```python
from build123d import *

# Parameters (mm, degrees)
SKETCH_R     = 14.5
PAD_DEPTH    = 35
SKETCH001_R  = 13.25
POCKET_DEPTH = 30
FILLET_R     = 1
FILLET001_R  = 1.2


with BuildPart() as part:
    # Sketch → Pad (new body)
    with BuildSketch(Plane.XY):
        Circle(SKETCH_R)
    extrude(amount=PAD_DEPTH)

    # Sketch001 (on Face3 of Pad) → Pocket (cut)
    with BuildSketch(Plane.XY.offset(35)):
        Circle(SKETCH001_R)
    extrude(amount=-POCKET_DEPTH, mode=Mode.SUBTRACT)

    # Fillet
    fillet_edges = [part.edges().sort_by_distance(p)[0] for p in [
        (-14.5, 0, 0),
    ]]
    fillet(fillet_edges, radius=FILLET_R)

    # Fillet001
    fillet001_edges = [part.edges().sort_by_distance(p)[0] for p in [
        (-14.5, 0, 35),
    ]]
    fillet(fillet001_edges, radius=FILLET001_R)


solid = part.part
```
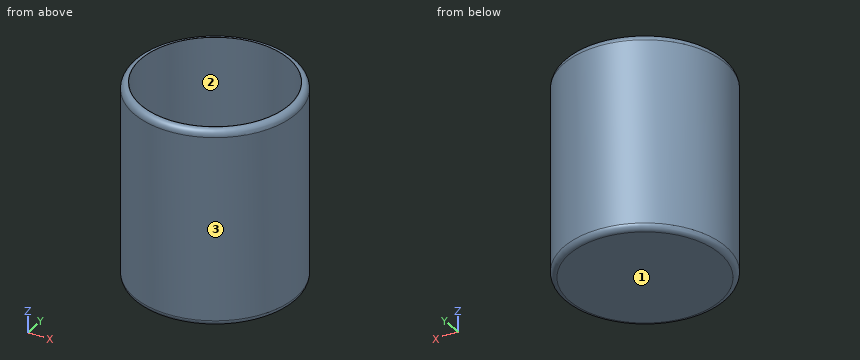
Part model, mm, in its own coordinate system. Face numbers are marked on the shaded views. Round coordinates to 2 decimals unless told otherwise and drop trailing zeros. Write each loop counter-clockwise with the first axis right and the second up, starting at its lowest first coordinate (ties: lowest second). Pieces come first, ordered by that corner, then holes.
Item 1: Probe L1, parallel to Y at x = 0, z = 19; L2, parallel to Z at x = -2.5, y = 12. List the from-to ranges inside material, lowest first.
Results:
L1: y = -14.5 to -13.25, 13.25 to 14.5
L2: z = 0 to 5
Item 2: Cut at A-A, the plane y = 0. Give the cut face in (x, z), plus the area to 3 significant figures.
Results:
outline: (-14.5, 1) arc R1 ccw to (-13.5, 0) - (13.5, 0) arc R1 ccw to (14.5, 1) - (14.5, 33.8) arc R1.2 ccw to (13.3, 35) - (13.25, 35) - (13.25, 5) - (-13.25, 5) - (-13.25, 35) - (-13.3, 35) arc R1.2 ccw to (-14.5, 33.8) - close
area: 219 mm2
Item 3: Cut at B-B, the plane z = 32. Give the cut face in (x, y).
Results:
outline: circle Ø29 at (0, 0); hole circle Ø26.5 at (0, 0)
Item 4: Cut at D-D, the plane z = 4.5. Give the cut face in (x, y), plus the area to 3 significant figures.
Results:
outline: circle Ø29 at (0, 0)
area: 661 mm2
Item 5: Two-plate mould, pull along X, no slides. Class the marked faces 1, 2 and 3: +X half, -X half, draft (parallel to the pull), parting line (faces both ways), or undercut.
Results:
face 1: draft
face 2: undercut
face 3: parting line
Item 6: Drop flat-ended pins along their axis: pin 1 Ø5 at (y, z) = (2.5, 21) entering from -X; pin 2 Ø4 at (y, z) = (-8.5, 7) entering from -X; pin 3 Ø4 at (x, y) = (0.5, 1.5) entering from +Z; pin 4 Ø12 at (y, z) = (-9.5, 22) entering from -X. Give the stop position or say it passes through.
Results:
pin 1: stops at x = -14.5
pin 2: stops at x = -12.96
pin 3: stops at z = 5
pin 4: stops at x = -14.07
